Design review of the part built by this model. Coordinates are the model's own, in mm. A direction names the side the tool comes from. Round coordinates to 2 decimals unless told otherwise and drop trailing zeros. Loops run counter-clockwise (first coordinate to the right, second up) from the corner with the lowest first, then second, coordinate; pieces in that order, holes last. Notation, with made-up numbers: M -4,-35 L 1,-35 A4 ccw 1,-30 Z; hole C -24.75,-1 d2. An arc over 180 degrees is marked long. One line per item, written item: value. Start each with the question number.
Item 1: We need section A-A (x = 0). Write out the cut boundary in (y, z) (3 decimals).
Item 2: We need section B-B (y = 0). Write out the cut boundary in (x, z) (3 decimals), then the cut area to 3 significant figures.
Item 3: Mouldability with a two-part tool opening along Y and no side actions: class faces 3 (the flat face through (18, 0, 23)), 4 (the flat face through (-3, -4, 2)), 5 (the cylindrical face through (17.98, 0.07, 6.4)) as released by +Y, released by -Y, zero draft, split by the parting line, or undercut.
Item 4: We need section D-D (z = 18.25). Write out the cut boundary in (x, y).
Item 5: For line 1 along X through (y, z) = (-3.5, 7.25); line 2 along Z through (x, y) = (-2, 2.5); line 3 along Y through (x, z) = (0, 1.25) (3 decimals), list the stretches that pass through material, from the lowest coordinate up.
Item 6: For faces 1 (the flat face through (-19.5, 0, 11)), 2 (the flat face through (16.5, 0, 13)), list the 3-axis set-ups (+Z, -Z, +X, -X, +Y, -Y) from which the entire face can be reached by the end or side of a thin tool; tool diameter is ignored.
Item 7: We need section C-C (z = 13.25). Write out the cut boundary in (x, y).
from build123d import *

# Parameters (mm, degrees)
SKETCH1_W           = 39
SKETCH1_H           = 8
BOSS_EXTRUDE1_DEPTH = 3
SKETCH2_W           = 3
SKETCH2_H           = 8
BOSS_EXTRUDE2_DEPTH = 20
SKETCH3_R           = 1.575
CUT_EXTRUDE1_DEPTH  = 40
SKETCH4_R           = 1.575
CUT_EXTRUDE2_DEPTH  = 3


with BuildPart() as part:
    # Sketch1 → Boss-Extrude1 (new body)
    with BuildSketch(Plane.XY):
        Rectangle(SKETCH1_W, SKETCH1_H)
    extrude(amount=BOSS_EXTRUDE1_DEPTH)

    # Sketch2 → Boss-Extrude2 (add)
    with BuildSketch(Plane.XY.offset(3)):
        with Locations((-18, 0)):
            Rectangle(SKETCH2_W, SKETCH2_H)
        with Locations((18, 0)):
            Rectangle(SKETCH2_W, SKETCH2_H)
    extrude(amount=BOSS_EXTRUDE2_DEPTH)

    # Sketch3 → Cut-Extrude1 (cut, through all)
    with BuildSketch(Plane.ZY.offset(19.5)):
        with Locations((18.025, 0)):
            Circle(SKETCH3_R)
        with Locations((7.975, 0)):
            Circle(SKETCH3_R)
    extrude(amount=-CUT_EXTRUDE1_DEPTH, mode=Mode.SUBTRACT)

    # Sketch4 → Cut-Extrude2 (cut)
    with BuildSketch(Plane.XY.offset(3)):
        Circle(SKETCH4_R)
    extrude(amount=-CUT_EXTRUDE2_DEPTH, mode=Mode.SUBTRACT)


solid = part.part
A:
1. outline: M -4,0 L -1.575,0 L -1.575,3 L -4,3 Z; M 1.575,0 L 4,0 L 4,3 L 1.575,3 Z
2. outline: M -19.5,0 L -1.575,0 L -1.575,3 L -16.5,3 L -16.5,6.4 L -19.5,6.4 Z; M -19.5,9.55 L -16.5,9.55 L -16.5,16.45 L -19.5,16.45 Z; M -19.5,19.6 L -16.5,19.6 L -16.5,23 L -19.5,23 Z; M 1.575,0 L 19.5,0 L 19.5,6.4 L 16.5,6.4 L 16.5,3 L 1.575,3 Z; M 16.5,9.55 L 19.5,9.55 L 19.5,16.45 L 16.5,16.45 Z; M 16.5,19.6 L 19.5,19.6 L 19.5,23 L 16.5,23 Z
2. area: 190 mm2
3. face 3: zero draft
3. face 4: released by -Y
3. face 5: undercut
4. outline: M -19.5,-4 L -16.5,-4 L -16.5,-1.56 L -19.5,-1.56 Z; M -19.5,1.56 L -16.5,1.56 L -16.5,4 L -19.5,4 Z; M 16.5,-4 L 19.5,-4 L 19.5,-1.56 L 16.5,-1.56 Z; M 16.5,1.56 L 19.5,1.56 L 19.5,4 L 16.5,4 Z
5. line 1: -19.5 to -16.5, 16.5 to 19.5
5. line 2: 0 to 3
5. line 3: -4 to -1.575, 1.575 to 4
6. face 1: +Z, -Z, -X, +Y, -Y
6. face 2: +Z, +Y, -Y
7. outline: M -19.5,-4 L -16.5,-4 L -16.5,4 L -19.5,4 Z; M 16.5,-4 L 19.5,-4 L 19.5,4 L 16.5,4 Z
